```python
from build123d import *

# Parameters (mm, degrees)
F1_DEPTH = 1.2
F2_R     = 0.3
F3_R     = 0.5


with BuildPart() as f1:
    # F0 (on Top) → F1 (new body)
    with BuildSketch(Plane.XY):
        with BuildLine():
            ThreePointArc((-0.75, 9.4703484624), (-6.4468984791, -6.9776428685), (9.5, 0))
            ThreePointArc((9.5, 0), (6.9776428685, 6.4468984791), (0.75, 9.4703484624))
            Line((0.75, 9.4703484624), (0.75, 7.9624057783))
            ThreePointArc((0.75, 7.9624057783), (1.1863210749, 7.9055818345), (1.61855899, 7.82326886))
            ThreePointArc((1.61855899, 7.82326886), (2.1373605639, 7.9807619738), (2.4946485572, 7.5729575551))
            ThreePointArc((2.4946485572, 7.5729575551), (3.3038970926, 7.2330724043), (4.0678951533, 6.8009704825))
            ThreePointArc((4.0678951533, 6.8009704825), (6.5863196722, 4.0875330208), (7.5, 0.5))
            ThreePointArc((7.5, 0.5), (-3.5875330208, -6.0863196722), (-4.0678951533, 6.8009704825))
            ThreePointArc((-4.0678951533, 6.8009704825), (-3.3038970926, 7.2330724043), (-2.4946485572, 7.5729575551))
            ThreePointArc((-2.4946485572, 7.5729575551), (-2.1373605639, 7.9807619738), (-1.61855899, 7.82326886))
            ThreePointArc((-1.61855899, 7.82326886), (-1.1863210749, 7.9055818345), (-0.75, 7.9624057783))
            Line((-0.75, 7.9624057783), (-0.75, 9.4703484624))
        make_face()
        with BuildLine():
            Line((-0.75, 5.9529404499), (-0.75, 7.9624057783))
            ThreePointArc((-0.75, 7.9624057783), (-1.1863210749, 7.9055818345), (-1.61855899, 7.82326886))
            ThreePointArc((-1.61855899, 7.82326886), (-1.5305745506, 7.6721619804), (-1.5, 7.5))
            ThreePointArc((-1.5, 7.5), (-2.0365767781, 7.0013396554), (-2.4946485572, 7.5729575551))
            ThreePointArc((-2.4946485572, 7.5729575551), (-3.3038970926, 7.2330724043), (-4.0678951533, 6.8009704825))
            Line((-4.0678951533, 6.8009704825), (-2.65, 5.3830753292))
            ThreePointArc((-2.65, 5.3830753292), (-1.7237130167, 5.7470699871), (-0.75, 5.9529404499))
        make_face()
        with BuildLine():
            ThreePointArc((1.61855899, 7.82326886), (1.1863210749, 7.9055818345), (0.75, 7.9624057783))
            Line((0.75, 7.9624057783), (0.75, 5.9529404499))
            ThreePointArc((0.75, 5.9529404499), (1.7237130167, 5.7470699871), (2.65, 5.3830753292))
            Line((2.65, 5.3830753292), (4.0678951533, 6.8009704825))
            ThreePointArc((4.0678951533, 6.8009704825), (3.3038970926, 7.2330724043), (2.4946485572, 7.5729575551))
            ThreePointArc((2.4946485572, 7.5729575551), (2.4986603446, 7.5365767781), (2.5, 7.5))
            ThreePointArc((2.5, 7.5), (1.8278380196, 7.0305745506), (1.61855899, 7.82326886))
        make_face()
    extrude(amount=F1_DEPTH)

    # F2
    f2_edges = [f1.edges().sort_by_distance(p)[0] for p in [
        (-0.75, 9.470348, 0.6),
        (0.75, 9.470348, 0.6),
    ]]
    fillet(f2_edges, radius=F2_R)

    # F3
    f3_edges = [f1.edges().sort_by_distance(p)[0] for p in [
        (-4.067895, 6.80097, 0.6),
        (4.067895, 6.80097, 0.6),
    ]]
    fillet(f3_edges, radius=F3_R)


solid = f1.part
```
Here's how the part is built. I have some questions about the finished solid (model axes, mm). A direction names the side the tool comes from. Coordinates: 2 decimals unless noted, no trailing zeros. Loops run counter-clockwise (first coordinate to the right, second up) from the corner with the lowest first, then second, coordinate; pieces in that order, holes last. Notation, with made-up numbers: (60, 85) - (71, 85) arc R14 cw to (71, 108) - close; hole circle Ø10 at (-23.5, 4.25). An arc over 180 degrees is marked (long way). Return JSON: item names as keys, results as strings. Group by question number.
Item 1: If we section it at C-C on z = 1: Write out the boundary of the cut face in (x, y).
Item 2: I need wall thicknesses on line 1 (X direction, y = 7.75, z = 0.3); line 2 (Y direction, x = 2, z = 0.3); line 3 (X direction, y = 6, z = 0.9). Which ranges of each line are inside material? Lowest first, please. Write a range as from..to.
Item 3: If we section it at D-D on x = -2: Write out the boundary of the cut face in (y, z).
Item 4: If we section it at B-B on y = 5: Write out the boundary of the cut face in (x, z), and give its area (3 significant figures).
Item 5: If we section it at A-A on x = 5: Write out the boundary of the cut face in (y, z), and give its area (3 significant figures).
Item 6: On a 3-axis mill with a long thin cutter (end or side, diameter ignored), from which of +Z, -Z, +X, -X, +Y, -Y can I reach the whole of each face in a straight line? I mean faces 3 (the face through (-2, 6, 0)), 4 (the face through (-0.75, 8, 1)), 5 (the face through (1.71, 5.75, 0.59)). Say none if no direction works.
Item 7: We'd pull the mould along X, two halves only. Please class faces 1 (the face through (-2, 6, 1.2)), 2 (the face through (-1.737, 5.743, 0.592)): +X half, -X half, draft (parallel to the pull), parting line (faces both ways), or undercut.
Calculated:
{
 "1": {"outline": "(-4.42, 6.56) arc R0.5 cw to (-3.77, 6.51) - (-2.65, 5.38) arc R6 cw to (-0.75, 5.95) - (-0.75, 9.14) arc R0.3 ccw to (-1.08, 9.44) arc R9.5 ccw (long way) to (1.08, 9.44) arc R0.3 ccw to (0.75, 9.14) - (0.75, 5.95) arc R6 cw to (2.65, 5.38) - (3.77, 6.51) arc R0.5 cw to (4.42, 6.56) arc R7.5 cw (long way) to start; hole circle Ø1 at (-2, 7.5); hole circle Ø1 at (2, 7.5)"},
 "2": {"line 1": "x = -5.49..-2.43, -1.57..-0.75, 0.75..1.57, 2.43..5.49", "line 2": "y = -9.29..-6.73, 5.66..7, 8..9.29", "line 3": "x = -7.37..-5.1, -3.27..-0.75, 0.75..3.27, 5.1..7.37"},
 "3": {"outline": "(-9.29, 0) - (-6.73, 0) - (-6.73, 1.2) - (-9.29, 1.2) - close; (5.66, 0) - (7, 0) - (7, 1.2) - (5.66, 1.2) - close; (8, 0) - (9.29, 0) - (9.29, 1.2) - (8, 1.2) - close"},
 "4": {"outline": "(-8.08, 0) - (-6, 0) - (-6, 1.2) - (-8.08, 1.2) - close; (6, 0) - (8.08, 0) - (8.08, 1.2) - (6, 1.2) - close", "area": "4.99 mm^2"},
 "5": {"outline": "(-8.08, 0) - (-5.09, 0) - (-5.09, 1.2) - (-8.08, 1.2) - close; (6.09, 0) - (8.08, 0) - (8.08, 1.2) - (6.09, 1.2) - close", "area": "5.97 mm^2"},
 "6": {"face 3": "-Z, +X, -X, +Y, -Y", "face 4": "+Z, -Z, +Y", "face 5": "+Z, -Z"},
 "7": {"face 1": "draft", "face 2": "undercut"}
}
